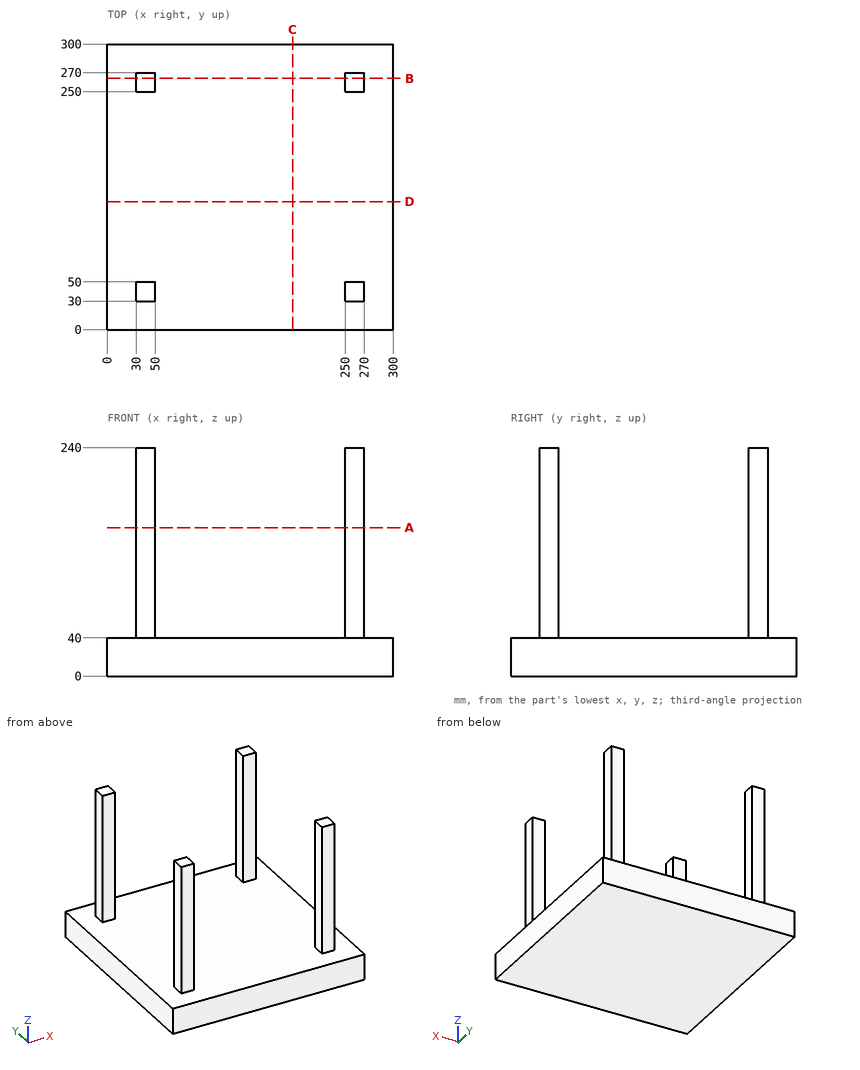
Geometry check sheet. Reference: drawing and pictorial views, mm from the part's lowest x, y, z. Coordinates: 2 decimals unless noted, no trailing zeros. Write each loop counter-clockwise with the first axis right and the second up, starting at its lowest first coordinate (ties: lowest second). Pieces come first, ordered by that corner, then holes. Notation, with made-up numbers: M -33.5,-12.75 L 17.5,-12.75 A26 cw 17.5,24.25 Z; hole C 27,-2.75 d4. An arc over 180 degrees is marked long. One line per question, with ' | ' between items.
1) Depth check by flat-ended pin: pin 1 Ø22 at (x, z) = (36.5, 102.5) entering from +Y; pin 2 Ø1 at (y, z) = (263.5, 163) entering from -X; pin 3 Ø5 at (x, y) = (53, 251) entering from -Z; pin 4 Ø22 at (x, z) = (255.5, 187) entering from -Y. Enter the tip coordinate at first touch or a pass-through.
Solutions:
pin 1: y = 270 | pin 2: x = 30 | pin 3: z = 0 | pin 4: y = 30
2) Material ranges on L1, parallel to Y at x = 34, z = 211.5; L2, parallel to Z at x = 188, y = 262.5, recorded low to high.
Solutions:
L1: 30 to 50, 250 to 270 | L2: 0 to 40
3) Sectioned sample at C-C on x = 194.5. Record the cut outline in (y, z).
Solutions:
outline: M 0,0 L 300,0 L 300,40 L 0,40 Z
4) Sectioned sample at B-B on y = 264. Record the cut outline in (x, z), then the cut area to 3 significant figures.
Solutions:
outline: M 0,0 L 300,0 L 300,40 L 270,40 L 270,240 L 250,240 L 250,40 L 50,40 L 50,240 L 30,240 L 30,40 L 0,40 Z | area: 20,000 mm^2
5) Sectioned sample at A-A on z = 156. Record the cut outline in (x, y), then the cut area to 3 significant figures.
Solutions:
outline: M 30,30 L 50,30 L 50,50 L 30,50 Z; M 30,250 L 50,250 L 50,270 L 30,270 Z; M 250,30 L 270,30 L 270,50 L 250,50 Z; M 250,250 L 270,250 L 270,270 L 250,270 Z | area: 1,600 mm^2
